Verification items for the finished model (mm, model axes). A direction names the side the tool comes from. Round coordinates to 2 decimals unless told otherwise and drop trailing zeros. Use CSV: the item, a comma, the result in double quotes.
Autodesk Inventor part; units mm, degrees
ref_plane "c1_XY" through (24.6126, 7.9057, 0) normal (0, 0, 1) x (1, 0, 0)
ref_plane "c1_YZ" through (24.6126, 7.9057, 0) normal (1, 0, 0) x (0, 1, 0)
ref_plane "c1_ZX" through (24.6126, 7.9057, 0) normal (0, 1, 0) x (0, 0, 1)
sketch "Sketch_8" plane through (0, 0, 0) normal (0, 0, 1) x (1, 0, 0)
  line L0 (24.6126, 0) -> (0, 0)
  line L1 (0, 0) -> (0, 8.9091)
  line L2 (0, 8.9091) -> (0.762, 9.671)
  line L3 (0.762, 9.671) -> (4.0386, 9.671)
  line L4 (4.0386, 9.671) -> (4.8006, 8.9091)
  line L5 (4.8006, 8.9091) -> (5.5626, 8.9091)
  line L6 (5.5626, 8.9091) -> (5.5626, 10.3759)
  line L7 (5.5626, 10.3759) -> (8.7363, 10.3759)
  line L8 (8.7363, 10.3759) -> (9.3142, 10.9537)
  line L9 (9.3142, 10.9537) -> (23.8506, 10.9537)
  line L10 (23.8506, 10.9537) -> (24.6126, 10.1918)
  line L11 (24.6126, 10.1918) -> (24.6126, 0)
  line L12 (24.6126, 0) -> (0, 0)
revolve "Revolution1" add sketch "Sketch_8" angle 360 about axis through (24.6126, 0, 0) along (1, 0, 0)
sketch "Sketch_15" plane through (0, 0, 0) normal (0, 0, 1) x (1, 0, 0)
  line L0 (40.4876, 0) -> (24.6126, 0)
  line L1 (24.6126, 0) -> (24.6126, 7.9057)
  line L2 (24.6126, 7.9057) -> (27.0002, 7.9057)
  line L3 (27.0002, 7.9057) -> (27.0002, 7.7279)
  arc A0 (27.0002, 7.7279) -> (27.8892, 6.839) centre (27.8892, 7.7279) ccw
  line L4 (27.8892, 6.839) -> (29.1719, 6.839)
  arc A1 (29.1719, 6.839) -> (29.7706, 7.0708) centre (29.1719, 7.7279) ccw
  line L5 (29.7706, 7.0708) -> (29.8005, 7.098)
  line L6 (29.8005, 7.098) -> (30.64, 7.9375)
  line L7 (30.64, 7.9375) -> (39.6481, 7.9375)
  line L8 (39.6481, 7.9375) -> (40.4876, 7.098)
  line L9 (40.4876, 7.098) -> (40.4876, 0)
  line L10 (40.4876, 0) -> (24.6126, 0)
revolve "Revolution2" add sketch "Sketch_15" angle 360 about axis through (40.4876, 0, 0) along (1, 0, 0)
thread "Thread1"
sketch "Sketch_9" plane through (40.4876, 0, 0) normal (1, 0, 0) x (0, 0, -1)
  line L0 (-21.9075, -43.815) -> (21.9075, -43.815)
  line L1 (21.9075, -43.815) -> (21.9075, 43.815)
  line L2 (21.9075, 43.815) -> (-21.9075, 43.815)
  line L3 (-21.9075, 43.815) -> (-21.9075, -43.815)
  line L4 (-4.7307, -21.9075) -> (4.7307, -21.9075)
  line L5 (4.7307, -21.9075) -> (4.7307, 21.9075)
  line L6 (4.7307, 21.9075) -> (-4.7307, 21.9075)
  line L7 (-4.7307, 21.9075) -> (-4.7307, -21.9075)
extrude "Extrusion1" cut sketch "Sketch_9" against normal blind 15.875
sketch "Sketch_13" plane through (0, 0, 0) normal (0, 0, 1) x (1, 0, 0)
  line L0 (23.7253, 0) -> (0, 0)
  line L1 (0, 0) -> (0, 3.9624)
  line L2 (0, 3.9624) -> (21.4376, 3.9624)
  line L3 (21.4376, 3.9624) -> (23.7253, 0)
  line L4 (23.7253, 0) -> (0, 0)
revolve "Revolution3" cut sketch "Sketch_13" angle 360 about axis through (23.7253, 0, 0) along (1, 0, 0)
sketch "Sketch_19" plane through (0, 0, 0) normal (0, 1, 0) x (-1, 0, 0)
  line L0 (-17.4752, 10.9537) -> (-17.4752, 0)
  line L1 (-17.4752, 0) -> (-22.04, 0)
  line L2 (-22.04, 0) -> (-22.04, 2.1565)
  line L3 (-22.04, 2.1565) -> (-22.2949, 10.3187)
  line L4 (-22.2949, 10.3187) -> (-22.9299, 10.9537)
  line L5 (-22.9299, 10.9537) -> (-17.4752, 10.9537)
  line L6 (-17.4752, 10.9537) -> (-17.4752, 0)
revolve "Revolution4" cut sketch "Sketch_19" angle 360 about axis through (17.4752, 0, 10.9537) along (0, 0, 1)
sketch "Sketch_24" plane through (0, 0, 0) normal (0, 0, 1) x (1, 0, 0)
  line L0 (5.5626, 0) -> (4.8006, 0)
  line L1 (4.4955, 10.2917) -> (5.4401, 9.3472)
  arc A0 (5.4401, 9.1676) -> (5.4401, 9.3472) centre (5.3503, 9.2574) ccw
  line L2 (5.4401, 9.1676) -> (5.1816, 8.9091)
  line L3 (5.1816, 8.9091) -> (4.8006, 8.9091)
  line L4 (4.8006, 8.9091) -> (4.8006, 8.655)
  line L5 (4.8006, 8.655) -> (5.5626, 8.655)
  line L6 (5.5626, 8.655) -> (5.5626, 9.512)
  line L7 (5.5626, 9.512) -> (4.6987, 10.3759)
  line L8 (4.6987, 10.3759) -> (4.4955, 10.3759)
  line L9 (4.4955, 10.3759) -> (4.4955, 10.2917)
revolve "Revolution5" add sketch "Sketch_24" angle 360 about axis through (5.5626, 0, 0) along (1, 0, 0)
sketch "Sketch_43" plane through (0, 0, 0) normal (0, 0, 1) x (1, 0, 0)
  circle A0 centre (33.3248, 0) radius 3.2004
extrude "Extrusion2" cut sketch "Sketch_43" along normal mid plane 14.1922
ref_plane "c1_XY" through (24.6126, 7.9057, 0) normal (0, 0, 1) x (1, 0, 0)
ref_plane "c1_YZ" through (24.6126, 7.9057, 0) normal (1, 0, 0) x (0, 1, 0)
ref_plane "c1_ZX" through (24.6126, 7.9057, 0) normal (0, 1, 0) x (0, 0, 1)
ref_plane "cc1_XY" through (24.6126, 0, 0) normal (0, 0, 1) x (1, 0, 0)
ref_plane "cc1_YZ" through (24.6126, 0, 0) normal (1, 0, 0) x (0, 1, 0)
ref_plane "cc1_ZX" through (24.6126, 0, 0) normal (0, 1, 0) x (0, 0, 1)
ref_plane "c2_XY" through (24.6126, -7.9057, 0) normal (0, 0, 1) x (1, 0, 0)
ref_plane "c2_YZ" through (24.6126, -7.9057, 0) normal (1, 0, 0) x (0, 1, 0)
ref_plane "c2_ZX" through (24.6126, -7.9057, 0) normal (0, 1, 0) x (0, 0, 1)
ref_plane "cc2_XY" through (27.0002, 0, 0) normal (0, 0, 1) x (1, 0, 0)
ref_plane "cc2_YZ" through (27.0002, 0, 0) normal (1, 0, 0) x (0, 1, 0)
ref_plane "cc2_ZX" through (27.0002, 0, 0) normal (0, 1, 0) x (0, 0, 1)
ref_plane "to_tube_XY" through (4.8006, 0, 0) normal (1, 0, 0) x (0, 0, -1)
ref_plane "to_tube_YZ" through (4.8006, 0, 0) normal (0, 0, -1) x (0, 1, 0)
ref_plane "to_tube_ZX" through (4.8006, 0, 0) normal (0, 1, 0) x (1, 0, 0)
ref_plane "to_nut_XY" through (24.6126, 0, 0) normal (1, 0, 0) x (0, 0, -1)
ref_plane "to_nut_YZ" through (24.6126, 0, 0) normal (0, 0, -1) x (0, 1, 0)
ref_plane "to_nut_ZX" through (24.6126, 0, 0) normal (0, 1, 0) x (1, 0, 0)
ref_plane "lovra1_XY" through (35.7124, 0, 0) normal (1, 0, 0) x (0, 0, -1)
ref_plane "lovra1_YZ" through (35.7124, 0, 0) normal (0, 0, -1) x (0, 1, 0)
ref_plane "lovra1_ZX" through (35.7124, 0, 0) normal (0, 1, 0) x (1, 0, 0)
ref_plane "lovra2_XY" through (35.7124, 7.874, 0) normal (1, 0, 0) x (0, 0, -1)
ref_plane "lovra2_YZ" through (35.7124, 7.874, 0) normal (0, 0, -1) x (0, 1, 0)
ref_plane "lovra2_ZX" through (35.7124, 7.874, 0) normal (0, 1, 0) x (1, 0, 0)
ref_plane "lovra3_XY" through (35.7124, -7.874, 0) normal (1, 0, 0) x (0, 0, -1)
ref_plane "lovra3_YZ" through (35.7124, -7.874, 0) normal (0, 0, -1) x (0, 1, 0)
ref_plane "lovra3_ZX" through (35.7124, -7.874, 0) normal (0, 1, 0) x (1, 0, 0)
ref_plane "to_pin_XY" through (33.3248, 0, 0) normal (0, 0, 1) x (1, 0, 0)
ref_plane "to_pin_YZ" through (33.3248, 0, 0) normal (1, 0, 0) x (0, 1, 0)
ref_plane "to_pin_ZX" through (33.3248, 0, 0) normal (0, 1, 0) x (0, 0, 1)
ref_plane "olen_XY" through (33.3248, 0, 0) normal (1, 0, 0) x (0, 0, -1)
ref_plane "olen_YZ" through (33.3248, 0, 0) normal (0, 0, -1) x (0, 1, 0)
ref_plane "olen_ZX" through (33.3248, 0, 0) normal (0, 1, 0) x (1, 0, 0)
ref_plane "thd1_XY" through (40.4876, 0, 7.9375) normal (1, 0, 0) x (0, 0, -1)
ref_plane "thd1_YZ" through (40.4876, 0, 7.9375) normal (0, 0, -1) x (0, 1, 0)
ref_plane "thd1_ZX" through (40.4876, 0, 7.9375) normal (0, 1, 0) x (1, 0, 0)
ref_plane "p1_XY" through (40.4876, 0, 4.7307) normal (1, 0, 0) x (0, 0, -1)
ref_plane "p1_YZ" through (40.4876, 0, 4.7307) normal (0, 0, -1) x (0, 1, 0)
ref_plane "p1_ZX" through (40.4876, 0, 4.7307) normal (0, 1, 0) x (1, 0, 0)
ref_plane "thd2_XY" through (40.4876, 0, -7.9375) normal (1, 0, 0) x (0, 0, -1)
ref_plane "thd2_YZ" through (40.4876, 0, -7.9375) normal (0, 0, -1) x (0, 1, 0)
ref_plane "thd2_ZX" through (40.4876, 0, -7.9375) normal (0, 1, 0) x (1, 0, 0)
ref_plane "p2_XY" through (40.4876, 0, -4.7307) normal (1, 0, 0) x (0, 0, -1)
ref_plane "p2_YZ" through (40.4876, 0, -4.7307) normal (0, 0, -1) x (0, 1, 0)
ref_plane "p2_ZX" through (40.4876, 0, -4.7307) normal (0, 1, 0) x (1, 0, 0)
ref_plane "port2_XY" through (40.4876, 0, 0) normal (1, 0, 0) x (0, 0, -1)
ref_plane "port2_YZ" through (40.4876, 0, 0) normal (0, 0, -1) x (0, 1, 0)
ref_plane "port2_ZX" through (40.4876, 0, 0) normal (0, 1, 0) x (1, 0, 0)
ref_plane "port_XY" through (17.4752, 0, 0) normal (0, 0, 1) x (1, 0, 0)
ref_plane "port_YZ" through (17.4752, 0, 0) normal (1, 0, 0) x (0, 1, 0)
ref_plane "port_ZX" through (17.4752, 0, 0) normal (0, 1, 0) x (0, 0, 1)
ref_plane "1_XY" through (24.6126, 0, 0) normal (1, 0, 0) x (0, 0, -1)
ref_plane "1_YZ" through (24.6126, 0, 0) normal (0, 0, -1) x (0, 1, 0)
ref_plane "1_ZX" through (24.6126, 0, 0) normal (0, 1, 0) x (1, 0, 0)
ref_plane "lovra21_XY" through (0, 0, 5.2705) normal (1, 0, 0) x (0, 0, -1)
ref_plane "lovra21_YZ" through (0, 0, 5.2705) normal (0, 0, -1) x (0, 1, 0)
ref_plane "lovra21_ZX" through (0, 0, 5.2705) normal (0, 1, 0) x (1, 0, 0)
ref_plane "lovra22_XY" through (0, 0, -5.2705) normal (1, 0, 0) x (0, 0, -1)
ref_plane "lovra22_YZ" through (0, 0, -5.2705) normal (0, 0, -1) x (0, 1, 0)
ref_plane "lovra22_ZX" through (0, 0, -5.2705) normal (0, 1, 0) x (1, 0, 0)
ref_plane "to_screw_XY" through (17.4752, 2.032, -6.0452) normal (0, 1, 0) x (1, 0, 0)
ref_plane "to_screw_YZ" through (17.4752, 2.032, -6.0452) normal (1, 0, 0) x (0, 0, -1)
ref_plane "to_screw_ZX" through (17.4752, 2.032, -6.0452) normal (0, 0, -1) x (0, 1, 0)
ref_plane "to_mounting_bracket_XY" through (24.6126, 0, 0) normal (1, 0, 0) x (0, 0, -1)
ref_plane "to_mounting_bracket_YZ" through (24.6126, 0, 0) normal (0, 0, -1) x (0, 1, 0)
ref_plane "to_mounting_bracket_ZX" through (24.6126, 0, 0) normal (0, 1, 0) x (1, 0, 0)
properties part number "04P0010_rear_head"
1) Thickness scan on probe 1 along Z at (x, y) = (5, -6); probe 2 along X at (y, z) = (3.75, 9); probe 3 along Z at (x, y) = (3, -0.5). Record the ranges inside material, lowest first. Write a range as [from, to].
Returned:
probe 1,"z = [-8.09, -7.73], [-6.59, 6.59], [7.73, 8.09]"
probe 2,"x = [5.04, 5.32], [5.56, 14.51], [20.44, 24.61]"
probe 3,"z = [-9.66, -3.93], [3.93, 9.66]"
2) Mould release check, pull along Z, two halves, no side actions. Record for faces 4 (the face through (4.994, -1.931, -8.697)), 5 (the face through (28.54, -6.84, 0.07)), 6 (the face through (0, 2, -4)): +Z half, -Z half, draft (parallel to the pull), parting line (faces both ways), or undercut.
Returned:
face 4,"undercut"
face 5,"parting line"
face 6,"draft"
3) Gauge pin test, flat ends, axial feed: pin 1 Ø1.4 at (y, z) = (-7.5, -1) entering from +X; pin 2 Ø4 at (x, y) = (36, 7) entering from -Z; pin 3 Ø12 at (x, y) = (14, 7.5) entering from -Z; pin 4 Ø6 at (x, z) = (19, -8) entering from +Y. Record the tip position at first contact, or that the pin passes through.
Returned:
pin 1,"stops at x = 40.49"
pin 2,"stops at z = -4.73"
pin 3,"stops at z = -10.85"
pin 4,"stops at y = 9.75"
4) Access from +Z, -Z, +X, -X, +Y, -Y to the whole of each face (thin tool, end or side, straight path). Record for faces 1 (the face through (29.946, 7.243, -0.074)), 2 (the face through (29.946, -7.243, 0.074)), 3 (the face through (7.172, -10.366, 0.456)).
Returned:
face 1,"+Y"
face 2,"-Y"
face 3,"-X"
5) Cross-section at A-A, the plane y = 1.25. Count the separate pieces of the cut face and the enclosed holes in it, then the cut area to 3 significant figures.
Returned:
separate pieces,"3"
enclosed holes,"0"
area,"376 mm²"
